The listing builds one solid part. Answer for the finished solid, in the listing's coordinates (mm). A direction names the side the tool comes from. Give positions to 0.01 mm unless a question says otherwise; leave off trailing zeros. Write each loop counter-clockwise with the first axis right and the second up, starting at its lowest first coordinate (ties: lowest second). Pieces come first, ordered by that corner, then holes. Notation, with made-up numbers: M -28.5,68 L 28.5,68 A23 cw 28.5,101 Z; hole C -38,6.5 d6. An arc over 180 degrees is marked long. Return JSON: item names as keys, results as strings.
Autodesk Inventor part; units mm, degrees
ref_plane "YZ Plane" through (0, 0, 0) normal (1, 0, 0) x (0, 1, 0)
ref_plane "XZ Plane" through (0, 0, 0) normal (0, 1, 0) x (-1, 0, 0)
ref_plane "XY Plane" through (0, 0, 0) normal (0, 0, 1) x (1, 0, 0)
sketch "Sketch1" plane through (0, 0, 0) normal (0, 1, 0) x (-1, 0, 0)
  line L0 (-7.25, 7.25) -> (7.25, 7.25)
  line L1 (7.25, 7.25) -> (7.25, -7.25)
  line L2 (7.25, -7.25) -> (-7.25, -7.25)
  line L3 (-7.25, -7.25) -> (-7.25, 7.25)
  line L4 (-7.25, 7.25) -> (7.25, -7.25) construction
  line L5 (7.25, 7.25) -> (-7.25, -7.25) construction
  point P0 (0, 0)
  dimension "d0" = 14.5
  dimension "d1" = 14.5
extrude "Extrusion1" add sketch "Sketch1" along normal blind 76.2
sketch "Sketch2" plane through (0, 76.2, 0) normal (0, 1, 0) x (1, 0, 0)
  line L0 (10, -10) -> (-10, -10)
  line L1 (-10, -10) -> (-10, 10)
  line L2 (-10, 10) -> (10, 10)
  line L3 (10, 10) -> (10, -10)
  line L4 (10, -10) -> (-10, 10) construction
  line L5 (-10, -10) -> (10, 10) construction
  point P0 (0, 0)
  dimension "d4" = 20
  dimension "d5" = 20
extrude "Extrusion2" add sketch "Sketch2" along normal blind 5
sketch "Sketch3" plane through (0, 81.2, 0) normal (0, 1, 0) x (1, 0, 0)
  line L0 (7.5, -7.5) -> (-7.5, -7.5)
  line L1 (-7.5, -7.5) -> (-7.5, 7.5)
  line L2 (-7.5, 7.5) -> (7.5, 7.5)
  line L3 (7.5, 7.5) -> (7.5, -7.5)
  line L4 (7.5, -7.5) -> (-7.5, 7.5) construction
  line L5 (-7.5, -7.5) -> (7.5, 7.5) construction
  line L6 (10, -10) -> (-10, -10)
  line L7 (-10, -10) -> (-10, 10)
  line L8 (-10, 10) -> (10, 10)
  line L9 (10, 10) -> (10, -10)
  line L10 (10, -10) -> (-10, 10) construction
  line L11 (-10, -10) -> (10, 10) construction
  point P0 (0, 0)
  dimension "d8" = 15
  dimension "d9" = 15
extrude "Extrusion3" add sketch "Sketch3" along normal blind 76.2
sketch "Sketch4" plane through (10, 76.2, 10) normal (1, 0, 0) x (0, 0, -1)
  line L0 (20, 0) -> (20, 81.2)
  line L1 (15, 81.2) -> (15, 0)
  line L2 (0, 0) -> (20, 0)
  line L3 (15, 81.2) -> (13, 81.2)
  line L4 (17.5, 81.2) -> (2.5, 81.2)
  line L5 (13, 81.2) -> (13, 0)
  line L6 (13, 0) -> (15, 0)
  line L7 (20, 81.2) -> (0, 81.2)
  point P0 (10, -76.2)
  dimension "d12" = 2
extrude "Extrusion4" add sketch "Sketch4" along normal blind 10 contours L2 L5 L3 L1
sketch "Sketch5" plane through (10, 76.2, -3) normal (0, 0, 1) x (1, 0, 0)
  line L0 (0, 81.2) -> (10, 81.2)
  line L1 (10, 81.2) -> (8, 81.2)
  line L2 (8, 81.2) -> (8, 0)
  line L3 (8, 0) -> (10, 0)
  line L4 (10, 0) -> (10, 81.2)
  point P0 (-10, -76.2)
  dimension "d15" = 2
extrude "Extrusion5" add sketch "Sketch5" along normal blind 8
sketch "Sketch6" plane through (20, 76.2, 10) normal (1, 0, 0) x (0, 0, -1)
  line L0 (5, 81.2) -> (3, 81.2)
  line L1 (3, 81.2) -> (3, 0)
  line L2 (3, 0) -> (5, 0)
  line L3 (5, 0) -> (5, 81.2)
  point P0 (10, -76.2)
  dimension "d18" = 2
extrude "Extrusion6" add sketch "Sketch6" against normal blind 4
sketch "Sketch7" plane through (0, 76.2, 0) normal (0, -1, 0) x (1, 0, 0)
  line L0 (10, -5) -> (20, -5)
  line L1 (20, -5) -> (20, 7)
  line L2 (20, 7) -> (10, 7)
  line L3 (10, 7) -> (10, -5)
  point P0 (0, 0)
extrude "Extrusion7" cut sketch "Sketch7" against normal through all
sketch "Sketch8" plane through (7.25, 0, -7.25) normal (0, 0, -1) x (-1, 0, 0)
  line L0 (0, 0) -> (0, 76.2)
  line L1 (0, 0) -> (0, 76.2)
  line L2 (0, 38.1) -> (14.5, 38.1)
  line L3 (14.5, 38.1) -> (14.5, 0)
  line L4 (14.5, 0) -> (0, 0)
  line L5 (0, 0) -> (0, 38.1)
  point P0 (7.25, 0)
extrude "Extrusion8" cut sketch "Sketch8" against normal through all
sketch "Sketch9" plane through (10, 76.2, -10) normal (0, 0, -1) x (-1, 0, 0)
  line L0 (0, 0) -> (0, 20)
  line L1 (0, 0) -> (0, 81.2)
  line L2 (0, 20) -> (20, 20)
  line L3 (20, 20) -> (20, 81.2)
  line L4 (20, 81.2) -> (0, 81.2)
  line L5 (0, 81.2) -> (0, 20)
  point P0 (10, -76.2)
  dimension "d25" = 20
extrude "Extrusion9" cut sketch "Sketch9" against normal through all
sketch "Sketch10" plane through (-10, 96.2, -10) normal (0, 1, 0) x (1, 0, 0)
  line L0 (17.5, -2.5) -> (2.5, -2.5)
  line L1 (2.5, -2.5) -> (2.5, -17.5)
  line L2 (2.5, -17.5) -> (17.5, -17.5)
  line L3 (17.5, -17.5) -> (17.5, -2.5)
  point P0 (10, -10)
extrude "Extrusion10" add sketch "Sketch10" against normal blind 15
sketch "Sketch11" plane through (10, 76.2, 10) normal (1, 0, 0) x (0, 0, -1)
  point P0 (10, -76.2)
sketch "Sketch12" plane through (-10, 76.2, -10) normal (-1, 0, 0) x (0, 0, 1)
  line L0 (0, 0) -> (0, 20)
  line L1 (20, 0) -> (20, 20)
  line L2 (20, 10) -> (15, 10)
  line L3 (0, 10) -> (5, 10)
  line L4 (20, 20) -> (23, 20)
  line L5 (23, 20) -> (23, 0)
  line L6 (23, 0) -> (20, 0)
  line L7 (20, 0) -> (20, 20)
  line L8 (0, 20) -> (-3, 20)
  line L9 (-3, 20) -> (-3, 0)
  line L10 (-3, 0) -> (0, 0)
  line L11 (0, 0) -> (0, 20)
  point P0 (10, -76.2)
  dimension "d30" = 5
  dimension "d31" = 5
  dimension "d32" = 3
  dimension "d33" = 3
extrude "Extrusion11" add sketch "Sketch12" against normal blind 20
sketch "Sketch13" plane through (-10, 76.2, -13) normal (-1, 0, 0) x (0, 0, 1)
  line L0 (20.25, 0) -> (5.75, 0)
  line L1 (0, 20) -> (8, 20)
  line L2 (8, 20) -> (8, 0)
  line L3 (8, 0) -> (0, 0)
  line L4 (0, 0) -> (0, 20)
  line L5 (26, 20) -> (18, 20)
  line L6 (18, 20) -> (18, 0)
  line L7 (18, 0) -> (26, 0)
  line L8 (26, 0) -> (26, 20)
  point P0 (13, -76.2)
  dimension "d36" = 8
  dimension "d37" = 8
extrude "Extrusion12" add sketch "Sketch13" along normal blind 25 contours L0 L6 L5 L8 L7
sketch "Sketch14" plane through (-10, 76.2, 5) normal (0, 0, -1) x (-1, 0, 0)
  line L0 (0, 20) -> (0, 0)
  line L1 (0, 10) -> (20, 10)
  circle A0 centre (20, 10) radius 3.75
  point P0 (-10, -76.2)
  dimension "d40" = 20
  dimension "d41" = 7.5
sketch "Sketch15" plane through (-10, 76.2, -13) normal (-1, 0, 0) x (0, 0, 1)
  point P0 (13, -76.2)
extrude "Extrusion13" add sketch "Sketch14" along normal blind 18
sketch "Sketch16" plane through (-10, 76.2, -13) normal (0, 0, -1) x (-1, 0, 0)
  point P0 (-10, -76.2)
properties part number "BearingEndCap"
Item 1: A cutting plane is placed at A-A, the plane z = 1.5. Write down the section's boundary in (x, y), plus the area to 3 significant figures.
Geometry results:
{"outline": "C -30,86.2 d7.5; M -10,76.2 L -7.25,76.2 L -7.25,38.1 L 7.25,38.1 L 7.25,76.2 L 10,76.2 L 10,96.2 L -10,96.2 Z", "area": "997 mm2"}
Item 2: A cutting plane is placed at C-C, the plane x = -30. Write down the section's boundary in (y, z).
Geometry results:
{"outline": "M 76.2,5 L 82.45,5 L 82.45,-13 L 89.95,-13 L 89.95,5 L 96.2,5 L 96.2,13 L 76.2,13 Z"}
Item 3: Which of the six approach directions +Z, -Z, +X, -X, +Y, -Y give full straight-line access (tool end or side, diameter ignored) to faces 5 (the flat face through (0, 57, -7.25)), 6 (the flat face through (0, 57, 7.25)), 7 (the flat face through (-10, 86, -4)), 8 (the flat face through (-22, 86, 5))?
Geometry results:
{"face 5": "-Z, +X, -X, -Y", "face 6": "+Z, +X, -X, -Y", "face 7": "-Z, +Y, -Y", "face 8": "-Z"}
Item 4: Given pin 1 Ø16 at (x, y) = (-2.5, 49.5) entering from +Z; pin 2 Ø10 at (x, z) = (-25.5, 2.5) entering from -Y; pin 3 Ø5.5 at (y, z) = (84.5, -1) entering from -X, each flat-ended and moving along its own axis, determine where each tip first touches the part or whether it passes through.
Geometry results:
{"pin 1": "stops at z = 7.25", "pin 2": "stops at y = 76.2", "pin 3": "stops at x = -33.75"}
Item 5: Find the intervals of material crossed by line 1 (X direction, y = 66, z = -1.75); line 2 (Y direction, x = -31, z = 9.5); line 3 (X direction, y = 94, z = -4.5), in increasing order.
Geometry results:
{"line 1": "x = -7.25 to 7.25", "line 2": "y = 76.2 to 96.2", "line 3": "x = -10 to 10"}
Item 6: A cutting plane is placed at D-D, the plane z = 11. Write down the section's boundary in (x, y).
Geometry results:
{"outline": "M -35,76.2 L 10,76.2 L 10,96.2 L -35,96.2 Z"}
Item 7: A cutting plane is placed at B-B, the plane y = 86.2. Write down the section's boundary in (x, z), plus the area to 3 significant figures.
Geometry results:
{"outline": "M -35,5 L -33.75,5 L -33.75,-13 L -26.25,-13 L -26.25,5 L -10,5 L -10,-13 L 10,-13 L 10,13 L -35,13 Z", "area": "855 mm2"}
Item 8: Determine the mould class of faces 1 (the flat face through (0, 86, -13)), 2 (the flat face through (-35, 86, 9)), 3 (the cylindrical face through (-29.19, 89.86, -3.87)), 4 (the flat face through (10, 86, 0)) for opening direction X: +X half, -X half, draft (parallel to the pull), parting line (faces both ways), or undercut.
Geometry results:
{"face 1": "draft", "face 2": "-X half", "face 3": "undercut", "face 4": "+X half"}
